```python
from build123d import *

# Parameters (mm, degrees)
SKETCH1_W           = 9.525
SKETCH1_H           = 9.525
SKETCH1_R           = 1.5
BOSS_EXTRUDE1_DEPTH = 6.35
SKETCH2_R           = 10
BOSS_EXTRUDE2_DEPTH = 13
SKETCH3_R           = 1.55
CUT_EXTRUDE1_DEPTH  = 11
SKETCH5_R           = 1.5
CUT_EXTRUDE2_DEPTH  = 10


with BuildPart() as part:
    # Sketch1 → Boss-Extrude1 (new body)
    with BuildSketch(Plane(origin=(0, 0, 0), x_dir=(1, 0, 0), z_dir=(0, 1, 0))):
        Rectangle(SKETCH1_W, SKETCH1_H)
        with Locations(Location((0, 0, 0), (0, 0, 270))):
            Circle(SKETCH1_R, mode=Mode.SUBTRACT)
    extrude(amount=BOSS_EXTRUDE1_DEPTH)

    # Sketch2 → Boss-Extrude2 (add)
    with BuildSketch(Plane.XZ):
        with Locations(Location((0, 0, 0), (0, 0, 90))):
            Circle(SKETCH2_R)
    extrude(amount=BOSS_EXTRUDE2_DEPTH)

    # Sketch3 → Cut-Extrude1 (cut)
    with BuildSketch(Plane.XZ.offset(13)):
        with Locations(Location((0, 0, 0), (0, 0, 270))):
            Circle(SKETCH3_R)
    extrude(amount=-CUT_EXTRUDE1_DEPTH, mode=Mode.SUBTRACT)

    # Sketch5 → Cut-Extrude2 (cut, symmetric)
    with BuildSketch(Plane.XY):
        with Locations((0, -6.5)):
            Circle(SKETCH5_R)
    extrude(amount=CUT_EXTRUDE2_DEPTH, both=True, mode=Mode.SUBTRACT)


solid = part.part
```
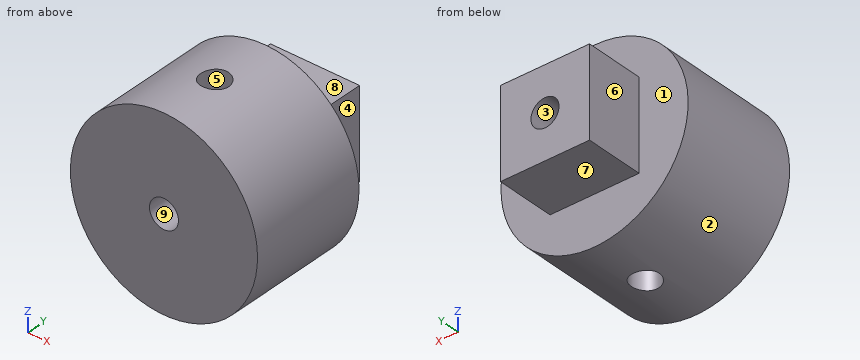
CAD build for the part. Positions are in the model's coordinates, mm. Face numbers are marked on the shaded views. A direction names the side the tool comes from. Round coordinates to 2 decimals unless told otherwise and drop trailing zeros. Loops run counter-clockwise (first coordinate to the right, second up) from the corner with the lowest first, then second, coordinate; pieces in that order, holes last. Notation, with made-up numbers: (-5, 4) - (1, 4) arc R11 ccw to (1, 16) - close; hole circle Ø6 at (55, 33). An arc over 180 degrees is marked (long way). Return JSON: item names as keys, results as strings. Group by question number.
Q1. Band-saw the part on C-C on z = -8.25. Give the cut face in (x, y), plus the area to 3 significant figures.
Q2. Band-saw the part on A-A on x = 0. Give the cut face in (y, z).
Q3. Two-plate mould, pull along X, no slides. Class the marked faces 1, 2, 3 and 4: +X half, -X half, draft (parallel to the pull), parting line (faces both ways), or undercut.
Q4. Band-saw the part on D-D on y = 1.5. Give the cut face in (x, z), plus the area to 3 significant figures.
Q5. Drill centre lines: line 1 along Y through (x, z) = (0, -7); line 2 along Y through (x, z) = (5, 4.5); line 3 along Y through (x, z) = (0, -3.25). Where is each one in solid material? Low to high. Write a range as [from, to].
Q6. Band-saw the part on B-B on y = -6.5. Give the cut face in (x, z), plus the area to 3 significant figures.
Q7. Tool access for the marked faces 5, 6, 7, 8 and 9: list every direction of +Z, -Z, +X, -X, +Y, -Y with a clear straight run to the whole face (end or side of a thin tool).
Q8. Flat gauge pins, fed straight in: pin 1 Ø1.8 at (x, z) = (0, 0) entering from +Y; pin 2 Ø1.9 at (x, y) = (1.5, 4) entering from +Z; pin 3 Ø5 at (x, y) = (2, 4) entering from -Z. Where does each tip first touch, or does it go through?
Solutions:
{
 "1": {"outline": "(-5.65, -13) - (5.65, -13) - (5.65, 0) - (-5.65, 0) - close; hole circle Ø3 at (0, -6.5)", "area": "140 mm^2"},
 "2": {"outline": "(-13, -10) - (-8, -10) - (-8, -1.55) - (-13, -1.55) - close; (-13, 1.55) - (-8, 1.55) - (-8, 10) - (-13, 10) - close; (-5, -10) - (0, -10) - (0, -4.76) - (6.35, -4.76) - (6.35, -1.5) - (0, -1.5) - (0, 1.5) - (6.35, 1.5) - (6.35, 4.76) - (0, 4.76) - (0, 10) - (-5, 10) - (-5, 1.55) - (-2, 1.55) - (-2, -1.55) - (-5, -1.55) - close"},
 "3": {"face 1": "draft", "face 2": "parting line", "face 3": "undercut", "face 4": "+X half"},
 "4": {"outline": "(-4.76, -4.76) - (4.76, -4.76) - (4.76, 4.76) - (-4.76, 4.76) - close; hole circle Ø3 at (0, 0)", "area": "83.7 mm^2"},
 "5": {"line 1": "y = [-13, -8], [-5, 0]", "line 2": "y = [-13, 0]", "line 3": "y = [-13, -8], [-5, 6.35]"},
 "6": {"outline": "(-1.5, -9.89) - (-1.5, -0.39) arc R1.55 cw to (-1.5, 0.39) - (-1.5, 9.89) arc R10 ccw to start; (1.5, -9.89) arc R10 ccw to (1.5, 9.89) - (1.5, 0.39) arc R1.55 cw to (1.5, -0.39) - close", "area": "254 mm^2"},
 "7": {"face 5": "+Z, -Z", "face 6": "+Z, -Z, -X, +Y", "face 7": "-Z, +X, -X, +Y", "face 8": "+Z, +X, -X, +Y", "face 9": "-Y"},
 "8": {"pin 1": "stops at y = 0", "pin 2": "stops at z = 4.76", "pin 3": "stops at z = -4.76"}
}
